from build123d import *

# Parameters (mm, degrees)
SKETCH1_R           = 2
SKETCH1_R_2         = 1.5
SKETCH1_R_3         = 2.25
BOSS_EXTRUDE1_DEPTH = 3.175


with BuildPart() as part:
    # Sketch1 → Boss-Extrude1 (new body)
    with BuildSketch(Plane(origin=(0, 0, 0), x_dir=(0, 0, -1), z_dir=(1, 0, 0))):
        with BuildLine():
            Line((-384.128639271, 211.620810697), (-360.186352931, 197.797725233))
            Line((-360.186352931, 197.797725233), (-360.186352931, 156.620810697))
            ThreePointArc((-360.186352931, 156.620810697), (-368.186352931, 148.620810697), (-376.186352931, 156.620810697))
            Line((-376.186352931, 156.620810697), (-376.186352931, 166.620810697))
            Line((-376.186352931, 166.620810697), (-409.095318274, 185.620810697))
            Line((-409.095318274, 185.620810697), (-479.479688809, 185.620810697))
            Line((-479.479688809, 185.620810697), (-505.186352931, 167.620810697))
            Line((-505.186352931, 167.620810697), (-505.186352931, 159.620810697))
            Line((-505.186352931, 159.620810697), (-535.186352931, 159.620810697))
            Line((-535.186352931, 159.620810697), (-535.186352931, 199.620810697))
            Line((-535.186352931, 199.620810697), (-523.186352931, 211.620810697))
            Line((-523.186352931, 211.620810697), (-384.128639271, 211.620810697))
        make_face()
        with Locations((-368.186352931, 156.620810697)):
            Circle(SKETCH1_R, mode=Mode.SUBTRACT)
        with Locations((-419.287503542, 205.620810697)):
            Circle(SKETCH1_R_2, mode=Mode.SUBTRACT)
        with Locations((-510.908050144, 194.119148631)):
            Circle(SKETCH1_R_3, mode=Mode.SUBTRACT)
        with Locations((-516.656718986, 176.534985115)):
            Circle(SKETCH1_R_3, mode=Mode.SUBTRACT)
        with Locations((-419.287503542, 191.620810697)):
            Circle(SKETCH1_R_2, mode=Mode.SUBTRACT)
        with Locations((-469.287503542, 205.620810697)):
            Circle(SKETCH1_R_2, mode=Mode.SUBTRACT)
        with Locations((-469.287503542, 191.620810697)):
            Circle(SKETCH1_R_2, mode=Mode.SUBTRACT)
        with Locations((-444.287503542, 205.620810697)):
            Circle(SKETCH1_R_2, mode=Mode.SUBTRACT)
        with Locations((-444.287503542, 191.620810697)):
            Circle(SKETCH1_R_2, mode=Mode.SUBTRACT)
    extrude(amount=BOSS_EXTRUDE1_DEPTH)


solid = part.part
CAD build for the part. Positions are in the model's coordinates, mm. A direction names the side the tool comes from. Give positions to 0.01 mm unless a question says otherwise; leave off trailing zeros. Write each loop counter-clockwise with the first axis right and the second up, starting at its lowest first coordinate (ties: lowest second). Pieces come first, ordered by that corner, then holes. Notation, with made-up numbers: (64.25, 45.5) - (94.25, 45.5) arc R8 ccw to (94.25, 55.5) - close; hole circle Ø5 at (8, -31.5). An arc over 180 degrees is marked (long way). Answer as CSV lines item,"result".
Q1. Pull direction Y, two halves, no side cores. Call faces 4 (the face through (1.57, 176.75, 492.15)), 5 (the face through (1.57, 177.21, 514.51)), 6 (the face through (2, 211.621, 455)): released by +Y, released by -Y, zero draft, split by the parting line, or undercut.
Result set:
face 4,"released by -Y"
face 5,"undercut"
face 6,"released by +Y"
Q2. Drill centre lines: line 1 (Y direction, x = 1.8, z = 511); line 2 (Z direction, x = 0.95, y = 166.5); line 3 (Y direction, x = 1.4, z = 434.5). Where is each one in solid material? Low to high. Write a range as from..to.
Result set:
line 1,"159.62..191.87, 196.37..211.62"
line 2,"360.19..376.19, 505.19..535.19"
line 3,"185.62..211.62"
Q3. Band-saw the part on A-A (x = 2). State how many separate pieces and enclosed holes the cut face has, and give its area (3 significant figures).
Result set:
separate pieces,"1"
enclosed holes,"9"
area,"6,110 mm²"
Q4. Band-saw the part on D-D (z = 481.5). Give the cut face in (x, y) (3 decimals), and give its area (3 significant figures).
Result set:
outline,"(0, 184.206) - (3.175, 184.206) - (3.175, 211.621) - (0, 211.621) - close"
area,"87.0 mm²"
Q5. 3-axis set-ups, long thin cutter, end or side, ignore diameter. For faces 1 (the face through (1.565, 191.923, 511.396)), 2 (the face through (1.565, 175.988, 392.41)), 3 (the face through (2, 159.621, 520)): which of +Z, -Z, +X, -X, +Y, -Y reach the whole face in a straight line?
Result set:
face 1,"+X, -X"
face 2,"+X, -X, -Y"
face 3,"+Z, +X, -X, -Y"
Q6. Band-saw the part on B-B (y = 171). Give the cut face in (x, z) (3 decimals), and give its area (3 significant figures).
Result set:
outline,"(0, 360.186) - (3.175, 360.186) - (3.175, 383.771) - (0, 383.771) - close; (0, 500.36) - (3.175, 500.36) - (3.175, 535.186) - (0, 535.186) - close"
area,"185 mm²"
Q7. Band-saw the part on C-C (z = 435). Give the cut face in (x, y) (3 decimals), and give its area (4 significant figures).
Result set:
outline,"(0, 185.621) - (3.175, 185.621) - (3.175, 211.621) - (0, 211.621) - close"
area,"82.55 mm²"
